```python
from build123d import *

# Parameters (mm, degrees)
F0_W     = 7
F0_H     = 52
F0_R     = 2
F1_DEPTH = 5
F0_W_2   = 33
F0_W_3   = 29
F0_H_2   = 47
F2_DEPTH = 35
F3_DEPTH = 5
F4_R     = 5
F5_R     = 2


with BuildPart() as f1:
    # F0 (on Top) → F1 (new body)
    with BuildSketch(Plane.XY):
        with Locations((-20, 0)):
            Rectangle(F0_W, F0_H)
        with Locations((-20, 8.5)):
            Circle(F0_R, mode=Mode.SUBTRACT)
    extrude(amount=F1_DEPTH)

    # F0 (on Top) → F2 (join)
    with BuildSketch(Plane.XY):
        Rectangle(F0_W_2, F0_H)
        Rectangle(F0_W_3, F0_H_2, mode=Mode.SUBTRACT)
    extrude(amount=F2_DEPTH)

    # F0 (on Top) → F3 (join)
    with BuildSketch(Plane.XY):
        with Locations((20, 0)):
            Rectangle(F0_W, F0_H)
        with Locations((20, 8.5)):
            Circle(F0_R, mode=Mode.SUBTRACT)
    extrude(amount=F3_DEPTH)

    # F4
    f4_edges = [f1.edges().sort_by_distance(p)[0] for p in [
        (-23.5, -26, 2.5),
        (23.5, -26, 2.5),
        (23.5, 26, 2.5),
        (-23.5, 26, 2.5),
    ]]
    fillet(f4_edges, radius=F4_R)

    # F5
    f5_edges = [f1.edges().sort_by_distance(p)[0] for p in [
        (-16.5, -26, 20),
        (16.5, -26, 20),
        (16.5, 26, 20),
        (-16.5, 26, 20),
    ]]
    fillet(f5_edges, radius=F5_R)


solid = f1.part
```
Source: CAD feature listing. Evaluate the final solid. Frame: model axes, mm. A direction names the side the tool comes from. Coordinates: 2 decimals unless noted, no trailing zeros. Write each loop counter-clockwise with the first axis right and the second up, starting at its lowest first coordinate (ties: lowest second). Pieces come first, ordered by that corner, then holes. Notation, with made-up numbers: (-2.75, 3) - (33.25, 3) arc R18 ccw to (33.25, 7) - close; hole circle Ø1 at (83, -22.75). An arc over 180 degrees is marked (long way). Answer as a JSON object with one key per item and string values.
Q1. Set-up query: faces 1 (the cylindrical face through (-15.93, 25.4, 20.21)), 2 (the flat face through (0, -23.5, 17)), 3 (the flat face through (-16, 0, 0)). Return all of +Z, -Z, +X, -X, +Y, -Y with unobstructed straight access to the full face (end or side cutting, diameter ignored); none if empty.
Ans:
{"face 1": "+Z, -X, +Y", "face 2": "+Z, -Z", "face 3": "-Z, +X, -X, +Y, -Y"}
Q2. Material intervals for line 1 (X direction, y = -6.5, z = 23.5); line 2 (Y direction, x = -1.5, z = 23.5); line 3 (X direction, y = 8, z = 2), sorted ascending. Write a range as [from, to].
Ans:
{"line 1": "x = [-16.5, -14.5], [14.5, 16.5]", "line 2": "y = [-26, -23.5], [23.5, 26]", "line 3": "x = [-23.5, -21.94], [-18.06, -14.5], [14.5, 18.06], [21.94, 23.5]"}
Q3. Draft query along Y for faces 4 (the cylindrical face through (15.9, -25.43, 20.21)), 5 (the flat face through (20, 0, 5)), 6 (the flat face through (-14.5, 0, 17)). Return one class per face: released by +Y, released by -Y, zero draft, split by the parting line, or undercut.
Ans:
{"face 4": "released by -Y", "face 5": "zero draft", "face 6": "undercut"}
Q4. Section query D-D, the plane y = 8.5. Output: boundary loops of the cut face in (x, z).
Ans:
{"outline": "(-23.5, 0) - (-22, 0) - (-22, 5) - (-23.5, 5) - close; (-18, 0) - (-14.5, 0) - (-14.5, 35) - (-16.5, 35) - (-16.5, 5) - (-18, 5) - close; (14.5, 0) - (18, 0) - (18, 5) - (16.5, 5) - (16.5, 35) - (14.5, 35) - close; (22, 0) - (23.5, 0) - (23.5, 5) - (22, 5) - close"}
Q5. First-contact query: pin 1 Ø17.5 at (y, z) = (10.5, 16) entering from -X; pin 2 Ø10.5 at (y, z) = (10, 13.5) entering from +X. Flat tips, straight axial feed; report the tip coordinate or a pass-through.
Ans:
{"pin 1": "stops at x = -16.5", "pin 2": "stops at x = 16.5"}
Q6. Section query A-A, the plane y = -12.5. Output: boundary loops of the cut face in (x, z).
Ans:
{"outline": "(-23.5, 0) - (-14.5, 0) - (-14.5, 35) - (-16.5, 35) - (-16.5, 5) - (-23.5, 5) - close; (14.5, 0) - (23.5, 0) - (23.5, 5) - (16.5, 5) - (16.5, 35) - (14.5, 35) - close"}
Q7. Section query C-C, the plane x = 8. Output: boundary loops of the cut face in (y, z), plus the area to 3 significant figures.
Ans:
{"outline": "(-26, 0) - (-23.5, 0) - (-23.5, 35) - (-26, 35) - close; (23.5, 0) - (26, 0) - (26, 35) - (23.5, 35) - close", "area": "175 mm2"}
Q8. Section query B-B, the plane z = 31. Output: boundary loops of the cut face in (x, y).
Ans:
{"outline": "(-16.5, -24) arc R2 ccw to (-14.5, -26) - (14.5, -26) arc R2 ccw to (16.5, -24) - (16.5, 24) arc R2 ccw to (14.5, 26) - (-14.5, 26) arc R2 ccw to (-16.5, 24) - close; hole (-14.5, -23.5) - (14.5, -23.5) - (14.5, 23.5) - (-14.5, 23.5) - close"}
